Verification items for this drawing (mm, ordinates from the low corner). Coordinates: 2 decimals unless noted, no trailing zeros. Order: outer loops, then holes, each group sorted by start corner. A loop starts at its lowest first (then second) coordinate and runs counter-clockwise, first axis right, second up. Notation, with made-up numbers: M 21.5,3 L 47.5,3 A21 ccw 47.5,14 Z; hole C -16,18.5 d5. An arc over 180 degrees is marked long. Return JSON: item names as keys, results as strings. Group by question number.
1. Material ranges on line 1 along Y through (x, z) = (5.3, 6.5); line 2 along Z through (x, y) = (5.25, 11); line 3 along Y through (x, z) = (3.75, 7.75) (1 decimal), recorded low to high.
2. Section check C-C, the plane z = 6.5. Record the cut outline in (x, y).
3. Section check B-B, the plane y = 5.85. Record the cut outline in (x, z).
4. Mould release check, pull along X, two halves, no side actions. Record for the marked faces 1, 2 and 3: +X half, -X half, draft (parallel to the pull), parting line (faces both ways), or undercut.
5. Section check D-D, the plane x = 3. Record the cut outline in (y, z), plus the area to 3 significant figures.
6. Section check A-A, the plane x = 5.3. Record the cut outline in (y, z).
7. Gauge pin test, flat end, axial feed: pin 1 (1 mm diameter, centred on x = 4, y = 4, fed in from -Z). Record the tip position at first contact, or that the pin passes through.
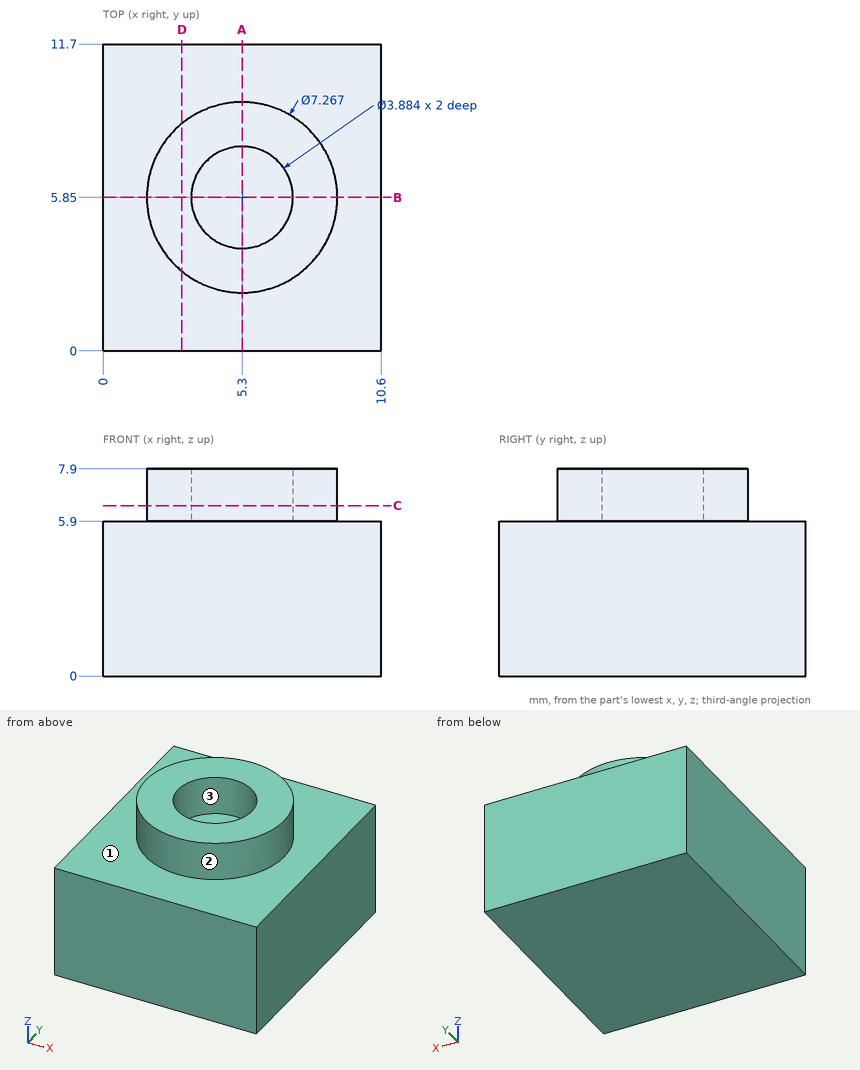
Answers follow:
{
 "1": {"line 1": "2.22 to 3.91, 7.79 to 9.48", "line 2": "0 to 5.9", "line 3": "2.6 to 4.7, 7 to 9.1"},
 "2": {"outline": "C 5.3,5.85 d7.27; hole C 5.3,5.85 d3.88"},
 "3": {"outline": "M 0,0 L 10.6,0 L 10.6,5.9 L 8.93,5.9 L 8.93,7.9 L 7.24,7.9 L 7.24,5.9 L 3.36,5.9 L 3.36,7.9 L 1.67,7.9 L 1.67,5.9 L 0,5.9 Z"},
 "4": {"face 1": "draft", "face 2": "parting line", "face 3": "undercut"},
 "5": {"outline": "M 0,0 L 11.7,0 L 11.7,5.9 L 8.66,5.9 L 8.66,7.9 L 3.04,7.9 L 3.04,5.9 L 0,5.9 Z", "area": "80.3 mm^2"},
 "6": {"outline": "M 0,0 L 11.7,0 L 11.7,5.9 L 9.48,5.9 L 9.48,7.9 L 7.79,7.9 L 7.79,5.9 L 3.91,5.9 L 3.91,7.9 L 2.22,7.9 L 2.22,5.9 L 0,5.9 Z"},
 "7": {"pin 1": "z = 0"}
}
